Geometry check sheet. Reference: the model listing, model coordinates, mm. A direction names the side the tool comes from. Round coordinates to 2 decimals unless told otherwise and drop trailing zeros. Loops run counter-clockwise (first coordinate to the right, second up) from the corner with the lowest first, then second, coordinate; pieces in that order, holes last. Notation, with made-up numbers: (75.25, 78) -> (97.25, 78) arc R23 cw to (97.25, 111) -> close; hole circle Ø6 at (18, 72.5). An arc over 180 degrees is marked (long way). Use one line per item in the form item = value.
from build123d import *

# Parameters (mm, degrees)
SKETCH_W     = 170
SKETCH_H     = 90
PAD_DEPTH    = 10
SKETCH001_R  = 2.5
PAD001_DEPTH = 10


with BuildPart() as part:
    # Sketch → Pad (new body)
    with BuildSketch(Plane.XY):
        with Locations((-60, 0)):
            Rectangle(SKETCH_W, SKETCH_H)
    extrude(amount=PAD_DEPTH)

    # Sketch001 (on Face6 of Pad) → Pad001 (join)
    with BuildSketch(Plane.XY.offset(10)):
        with Locations((-40, 0)):
            Circle(SKETCH001_R)
        Circle(SKETCH001_R)
        with Locations((-100, 0)):
            Circle(SKETCH001_R)
    extrude(amount=PAD001_DEPTH)


solid = part.part
1. Mould release check, pull along X, two halves, no side actions. Record for faces 3 (the flat face through (-145, -1, 5)), 4 (the flat face through (25, -1, 5)), 5 (the flat face through (-100, 0, 20)), 6 (the cylindrical face through (-97.615, 0.751, 14.93)): released by +X, released by -X, zero draft, split by the parting line, or undercut.
Return value:
face_3 = released by -X
face_4 = released by +X
face_5 = zero draft
face_6 = undercut
2. Section check B-B (x = 0). Record the boundary of the cut face in (y, z), then the cut area to 3 significant figures.
Return value:
outline = (-45, 0) -> (45, 0) -> (45, 10) -> (2.5, 10) -> (2.5, 20) -> (-2.5, 20) -> (-2.5, 10) -> (-45, 10) -> close
area = 950 mm2
3. Section check C-C (z = 18). Record the boundary of the cut face in (x, y), then the cut area to 3 significant figures.
Return value:
outline = circle Ø5 at (-100, 0); circle Ø5 at (-40, 0); circle Ø5 at (0, 0)
area = 58.9 mm2
4. Section check A-A (y = 0). Record the boundary of the cut face in (x, z).
Return value:
outline = (-145, 0) -> (25, 0) -> (25, 10) -> (2.5, 10) -> (2.5, 20) -> (-2.5, 20) -> (-2.5, 10) -> (-37.5, 10) -> (-37.5, 20) -> (-42.5, 20) -> (-42.5, 10) -> (-97.5, 10) -> (-97.5, 20) -> (-102.5, 20) -> (-102.5, 10) -> (-145, 10) -> close
5. Material ranges on line 1 along Z through (x, y) = (-58, -28); line 2 along Y through (x, z) = (1.5, 13.25), recorded low to high.
Return value:
line_1 = 0 to 10
line_2 = -2 to 2
6. Gauge pin test, flat end, axial feed: pin 1 (1 mm diameter, centred on x = -104.5, y = -17.5, fed in from +Z). Record the tip position at first contact, or that the pin passes through.
Return value:
pin_1 = 10
7. Section check D-D (x = -77). Record the boundary of the cut face in (y, z), then the cut area to 3 significant figures.
Return value:
outline = (-45, 0) -> (45, 0) -> (45, 10) -> (-45, 10) -> close
area = 900 mm2
8. Tool access check on faces 1 (the cylindrical face through (-37.69, -0.96, 14.93)), 2 (the flat face through (-61, 1, 0)). Record the directions out of +Z, -Z, +X, -X, +Y, -Y that give a thin tool (end or side, any length) a straight path to the whole face; none if there is none.
Return value:
face_1 = +Z
face_2 = -Z, +X, -X, +Y, -Y
